Input: part model. Units: mm. Frame: model coordinates. A direction names the side the tool comes from. Coordinates: 2 decimals unless noted, no trailing zeros. Order: outer loops, then holes, each group sorted by start corner. A loop starts at its lowest first (then second) coordinate and runs counter-clockwise, first axis right, second up. Notation, with made-up numbers: M 53,57.25 L 88,57.25 A31 cw 88,88.25 Z; hole C 76,89 d2. An arc over 180 degrees is marked long. Answer in a Markdown table with one row per item.
from build123d import *

# Parameters (mm, degrees)
SKETCH1_W           = 1568.45
SKETCH1_H           = 63.5
BOSS_EXTRUDE1_DEPTH = 63.5
SHELL1_T            = -6.35
SKETCH3_W           = 47.752
SKETCH3_H           = 44.45
CUT_EXTRUDE1_DEPTH  = 6.35


with BuildPart() as part:
    # Sketch1 → Boss-Extrude1 (new body)
    with BuildSketch(Plane.XY):
        with Locations((0, 31.75)):
            Rectangle(SKETCH1_W, SKETCH1_H)
    extrude(amount=BOSS_EXTRUDE1_DEPTH)

    # Shell1
    shell1_openings = [part.faces().sort_by_distance(p)[0] for p in [
        (0, 63.5, 31.75),
        (784.225, 31.75, 31.75),
    ]]
    offset(amount=SHELL1_T, openings=shell1_openings, kind=Kind.INTERSECTION)

    # Sketch3 → Cut-Extrude1 (cut)
    with BuildSketch(Plane.XY.offset(63.5)):
        with Locations((-753.999, 41.275)):
            Rectangle(SKETCH3_W, SKETCH3_H)
    extrude(amount=-CUT_EXTRUDE1_DEPTH, mode=Mode.SUBTRACT)


solid = part.part
1) Cut plane B-B, the plane z = 17. Output: boundary loops of the cut face in (x, y) (3 decimals).
Resolved:
| item | result |
|---|---|
| outline | M -784.225,0 L 784.225,0 L 784.225,6.35 L -777.875,6.35 L -777.875,63.5 L -784.225,63.5 Z |
2) Reachability of faces 1 (the face through (-8, 6.35, 31)), 2 (the face through (-11, 0, 31)) from +Z, -Z, +X, -X, +Y, -Y: full face, straight path, thin tool, end or side. Return the list, or none.
Resolved:
| item | result |
|---|---|
| face 1 | +X, +Y |
| face 2 | +Z, -Z, +X, -X, -Y |
3) Material intervals for probe 1 along Z at (x, y) = (-578, 29); probe 2 along X at (y, z) = (50, 60.5) (3 decimals), sorted ascending.
Resolved:
| item | result |
|---|---|
| probe 1 | z = 0 to 6.35, 57.15 to 63.5 |
| probe 2 | x = -784.225 to -777.875, -730.123 to 784.225 |
4) Mould query, pull axis Z, two halves, no side actions, for faces 3 (the face through (-11, 32, 63.5)), 4 (the face through (-8, 35, 6.35)), 5 (the face through (-4, 63.5, 3)). Classes: +Z half, -Z half, draft (parallel to the pull), parting line (faces both ways), or undercut.
Resolved:
| item | result |
|---|---|
| face 3 | +Z half |
| face 4 | undercut |
| face 5 | draft |
5) Cut plane C-C, the plane x = -479. Output: boundary loops of the cut face in (y, z).
Resolved:
| item | result |
|---|---|
| outline | M 0,0 L 63.5,0 L 63.5,6.35 L 6.35,6.35 L 6.35,57.15 L 63.5,57.15 L 63.5,63.5 L 0,63.5 Z |
6) Cut plane A-A, the plane y = 45. Output: boundary loops of the cut face in (x, z) (3 decimals), and give its area (3 significant figures).
Resolved:
| item | result |
|---|---|
| outline | M -784.225,0 L 784.225,0 L 784.225,6.35 L -777.875,6.35 L -777.875,63.5 L -784.225,63.5 Z; M -730.123,57.15 L 784.225,57.15 L 784.225,63.5 L -730.123,63.5 Z |
| area | 19,900 mm2 |
7) Contact query for flat-ended pins moving along their axis: pin 1 (7 mm diameter, centred on x = -758.5, z = 60.5, fed in from +Y); pin 2 (5 mm diameter, centred on x = 496.5, z = 24.5, fed in from +Y); pin 3 (4 mm diameter, centred on y = 9, z = 40, fed in from +X) (3 decimals). Output: stop coordinate, or through.
Resolved:
| item | result |
|---|---|
| pin 1 | stops at y = 19.05 |
| pin 2 | stops at y = 6.35 |
| pin 3 | stops at x = -777.875 |
